Check sheet for the modelled part. Datum: model origin and axes. Units: mm. Face numbers are marked on the shaded views. A direction names the side the tool comes from. Coordinates: 2 decimals unless noted, no trailing zeros. Order: outer loops, then holes, each group sorted by start corner. A loop starts at its lowest first (then second) coordinate and runs counter-clockwise, first axis right, second up. Notation, with made-up numbers: (26.5, 88.25) -> (37.5, 88.25) arc R38 ccw to (37.5, 127.25) -> close; hole circle Ø6 at (2.25, 14). An arc over 180 degrees is marked (long way). Put each result on its own line as item: value. Start each with the question number.
```python
from build123d import *

# Parameters (mm, degrees)
F1_DEPTH = 9
F2_R     = 5
F3_R     = 1.75
F4_DEPTH = 5.5


with BuildPart() as f1:
    # F0 (on Right) → F1 (new body)
    with BuildSketch(Plane.YZ):
        Polygon((17.2, 58.5), (17.2, 54), (19.6, 54), (19.6, 62), (-35.795717, 62), (0, 0), (19.6, 0), (19.6, 8), (17.2, 8), (17.2, 3.5), (15.5, 3.5), (15.5, 9.5), (7, 9.5), (7, 52.5), (15.5, 52.5), (15.5, 58.5), align=None)
        Polygon((0, 10), (-27.135463, 57), (0, 57), align=None, mode=Mode.SUBTRACT)
    extrude(amount=F1_DEPTH)

    # F2
    f2_edges = [f1.edges().sort_by_distance(p)[0] for p in [
        (4.5, 0, 57),
        (4.5, -27.135463, 57),
        (4.5, 0, 10),
    ]]
    fillet(f2_edges, radius=F2_R)

    # F3 (on face) → F4 (join)
    with BuildSketch(Plane(origin=(0, 0, 0), x_dir=(1, 0, 0), z_dir=(0, -0.866025, -0.5))):
        with BuildLine():
            Line((15.5, 63.795717), (9, 63.795717))
            Line((9, 63.795717), (9, 57.795717))
            Line((9, 57.795717), (15.5, 57.795717))
            ThreePointArc((15.5, 57.795717), (18.5, 60.795717), (15.5, 63.795717))
        make_face()
        with Locations((15.5, 60.795717)):
            Circle(F3_R, mode=Mode.SUBTRACT)
        with BuildLine():
            Line((15.5, 13.795717), (9, 13.795717))
            Line((9, 13.795717), (9, 7.795717))
            Line((9, 7.795717), (15.5, 7.795717))
            ThreePointArc((15.5, 7.795717), (18.5, 10.795717), (15.5, 13.795717))
        make_face()
        with Locations((15.5, 10.795717)):
            Circle(F3_R, mode=Mode.SUBTRACT)
    extrude(amount=-F4_DEPTH)


solid = f1.part
```
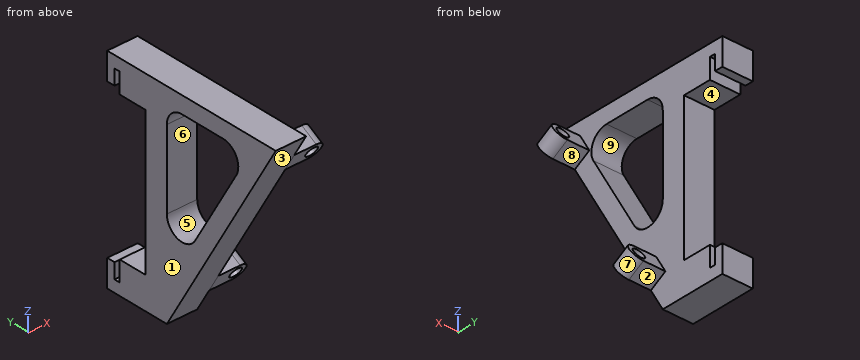
1) Gauge pin test, flat ends, axial feed: pin 1 (2.5 mm diameter, centred on y = -30.5, z = 53.5, fed in from -X); pin 2 (5 mm diameter, centred on x = 5, z = 5.5, fed in from -Y); pin 3 (12 mm diameter, centred on y = -5.5, z = 32, fed in from +X); pin 4 (2.5 mm diameter, centred on x = 3.5, y = -13.5, fed in from -Z). Record the tip position at first contact, or that the pin passes through.
2) Sectioned sample at C-C (x = 6). Record the boundary of the cut face in (y, z).
3) Mould release check, pull along Y, two halves, no side actions. Record for the marked faces 6, 7, 8 and 9: +Y half, -Y half, draft (parallel to the pull), parting line (faces both ways), or undercut.
4) Sectioned sample at B-B (z = 4.5). Record the boundary of the cut face in (x, y), plus the area to 3 significant figures.
5) Access from +Z, -Z, +X, -X, +Y, -Y to the whole of each face (thin tool, end or side, straight path). Record for the marked faces 1, 2, 3, 4 and 5.
6) Sectioned sample at A-A (y = 16.5). Record the boundary of the cut face in (x, z).
7) Scan lines: line 1 along Y through (x, z) = (6.25, 56.5); line 2 along Z through (x, y) = (4, 17); line 3 along Y through (x, z) = (4, 47). Record each from-to range of solid material in increasing order. Write a range as [from, to].
Entries:
1. pin 1: stops at x = 0
1. pin 2: stops at y = -4.62
1. pin 3: stops at x = 9
1. pin 4: stops at z = 21.22
2. outline: (-35.8, 62) -> (0, 0) -> (19.6, 0) -> (19.6, 8) -> (17.2, 8) -> (17.2, 3.5) -> (15.5, 3.5) -> (15.5, 9.5) -> (7, 9.5) -> (7, 52.5) -> (15.5, 52.5) -> (15.5, 58.5) -> (17.2, 58.5) -> (17.2, 54) -> (19.6, 54) -> (19.6, 62) -> close; hole (-22.81, 49.5) -> (-9.33, 26.16) arc R5 ccw to (0, 28.66) -> (0, 52) arc R5 ccw to (-5, 57) -> (-18.48, 57) arc R5 ccw to start
3. face 6: undercut
3. face 7: parting line
3. face 8: +Y half
3. face 9: undercut
4. outline: (0, -2.6) -> (9, -2.6) -> (9, 15.5) -> (0, 15.5) -> close; (0, 17.2) -> (9, 17.2) -> (9, 19.6) -> (0, 19.6) -> close
4. area: 184 mm2
5. face 1: +Z, -Z, -X, +Y, -Y
5. face 2: -Z, +X, +Y
5. face 3: -Z, +X, -X, -Y
5. face 4: +X, -X, +Y
5. face 5: +X, -X
6. outline: (0, 0) -> (9, 0) -> (9, 3.5) -> (0, 3.5) -> close; (0, 58.5) -> (9, 58.5) -> (9, 62) -> (0, 62) -> close
7. line 1: y = [-32.62, -20.65], [-2.82, 15.5], [17.2, 19.6]
7. line 2: z = [0, 3.5], [58.5, 62]
7. line 3: y = [-27.14, -21.36], [0, 7]
